Could you check a few things on this model? Use its own coordinates, in mm. A direction names the side the tool comes from. Coordinates: 2 decimals unless noted, no trailing zeros. Loops run counter-clockwise (first coordinate to the right, second up) from the corner with the lowest first, then second, coordinate; pieces in that order, holes last. Notation, with made-up numbers: (44.25, -23) -> (79.25, -23) arc R25 cw to (79.25, 5) -> close; hole circle Ø7 at (23.5, 40). An arc over 180 degrees is marked (long way). One line per question, with ' | ' between items. Start each with the question number.
(1) If we mould it in two halves opening along X, with no side actions, what happens to faces 1 (the face through (-78.5, 0, -24)), 2 (the face through (-63, 0, -2)), 3 (the face through (-1, 0, 0)), 4 (the face through (78.5, 0, -24))? For each: pulls with the +X half, pulls with the -X half, needs draft (parallel to the pull), parting line crosses it, or undercut.
(2) I'm going to push a flat-ended pin straight in: pin 1 Ø17.5 at (x, y) = (62.5, 0) entering from +Z. Where does the tip first touch, or does it pass through?
(3) Suppose I cut it at B-B (x = 65.5). Please give me the cut outline in (y, z), plus the area to 3 significant figures.
(4) If I drill on line 1 along Y through (x, z) = (62.5, -0.95); line 2 along Z through (x, y) = (-63, -5), over which ranges is the centre line in solid material (lowest first)?
(5) Which directions (+Z, -Z, +X, -X, +Y, -Y) give clear straight access to the entire face, cutting with the end or side of a thin tool? Please do faces 5 (the face through (-73.49, 0.48, -0.99)), 6 (the face through (1, -17.5, -24)).
(6) Suppose I cut it at A-A (x = -62.5). Please give me the cut outline in (y, z).
Autodesk Inventor part; units mm, degrees
ref_plane "YZ Plane" through (0, 0, 0) normal (1, 0, 0) x (0, 1, 0)
ref_plane "XZ Plane" through (0, 0, 0) normal (0, 1, 0) x (-1, 0, 0)
ref_plane "XY Plane" through (0, 0, 0) normal (0, 0, 1) x (1, 0, 0)
sketch "Sketch1" plane through (0, 0, 0) normal (0, 0, 1) x (1, 0, 0)
  line L0 (-78.5, 17.5) -> (78.5, 17.5)
  line L1 (78.5, 17.5) -> (78.5, -17.5)
  line L2 (78.5, -17.5) -> (-78.5, -17.5)
  line L3 (-78.5, -17.5) -> (-78.5, 17.5)
  point P0 (0, 0)
  point P1 (0, 17.5)
  point P2 (78.5, 0)
  dimension "d0" = 157
  dimension "d1" = 35
extrude "Extrusion1" add sketch "Sketch1" against normal blind 48
sketch "Sketch2" plane through (0, 0, 0) normal (0, 0, 1) x (1, 0, 0)
  circle A0 centre (-62.5, 0) radius 11
  circle A1 centre (62.5, 0) radius 11
  line L0 (-78.5, -17.5) -> (-78.5, 17.5)
  point P0 (0, 0)
  dimension "d4" = 22
  dimension "d5" = 22
  dimension "d6" = 125
  dimension "d7" = 16
extrude "Extrusion2" cut sketch "Sketch2" against normal blind 2
equation "\"d5\" = d4"
properties part number "Camera" material "Brass, Soft Yellow"
Checks:
1) face 1: pulls with the -X half | face 2: undercut | face 3: needs draft | face 4: pulls with the +X half
2) pin 1: stops at z = -2
3) outline: (-17.5, -48) -> (17.5, -48) -> (17.5, 0) -> (10.58, 0) -> (10.58, -2) -> (-10.58, -2) -> (-10.58, 0) -> (-17.5, 0) -> close | area: 1,640 mm^2
4) line 1: y = -17.5 to -11, 11 to 17.5 | line 2: z = -48 to -2
5) face 5: +Z | face 6: +Z, -Z, +X, -X, -Y
6) outline: (-17.5, -48) -> (17.5, -48) -> (17.5, 0) -> (11, 0) -> (11, -2) -> (-11, -2) -> (-11, 0) -> (-17.5, 0) -> close
